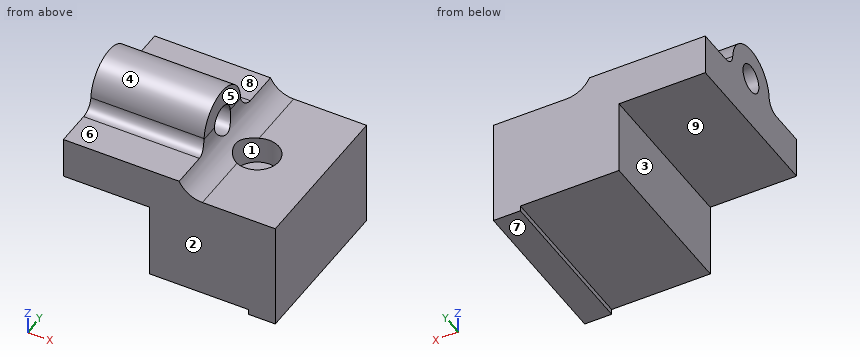
from build123d import *

# Parameters (mm, degrees)
PAD003_DEPTH         = 30
POCKET001_DEPTH      = 21.001
POCKET001_DEPTH_BACK = 18.286158
SKETCH010_R          = 2.6
POCKET002_DEPTH      = 21.001
POCKET002_DEPTH_BACK = 18.286158
SKETCH011_R          = 4
POCKET003_DEPTH      = 5
POCKET003_DEPTH_BACK = 100


with BuildPart() as part:
    # Sketch008 → Pad003 (new body)
    with BuildSketch(Plane.XZ):
        with BuildLine():
            Line((-16, 15), (0, 15))
            Line((0, 15), (0, 1))
            Line((0, 1), (18.285158, 1))
            Line((18.285158, 1), (18.285158, 0))
            Line((18.285158, 0), (23.285158, 0))
            Line((23.285158, 0), (23.285158, 20))
            Line((23.285158, 20), (9.7625, 20))
            ThreePointArc((5, 24.7625), (6.394904, 21.394904), (9.7625, 20))
            Line((5, 24.7625), (5, 30.6))
            Line((5, 30.6), (-16, 30.6))
            Line((-16, 30.6), (-16, 15))
        make_face()
    extrude(amount=PAD003_DEPTH)

    # Sketch009 (on Face1 of Pad003) → Pocket001 (cut, two sides)
    with BuildSketch(Plane(origin=(5, 0, 0), x_dir=(0, 0, 1), z_dir=(1, 0, 0))) as pocket001_sk:
        with BuildLine():
            ThreePointArc((24.943511, 9.009841), (30.6, 15), (24.943511, 20.990159))
            ThreePointArc((22.698592, 23.367503), (23.348515, 21.732615), (24.943511, 20.990159))
            Line((22.698592, 23.367503), (22.698592, 35))
            Line((22.698592, 35), (35.6, 35))
            Line((35.6, 35), (35.6, -5))
            Line((35.6, -5), (22.698592, -5))
            Line((22.698592, -5), (22.698592, 6.632497))
            ThreePointArc((24.943511, 9.009841), (23.348515, 8.267384), (22.698592, 6.632497))
        make_face()
    extrude(amount=-POCKET001_DEPTH, mode=Mode.SUBTRACT)
    extrude(pocket001_sk.sketch, amount=POCKET001_DEPTH_BACK, mode=Mode.SUBTRACT)

    # Sketch010 (on Face1 of Pocket001) → Pocket002 (cut, two sides)
    with BuildSketch(Plane(origin=(5, 0, 0), x_dir=(0, 0, 1), z_dir=(1, 0, 0))) as pocket002_sk:
        with Locations((24.6, 15)):
            Circle(SKETCH010_R)
    extrude(amount=-POCKET002_DEPTH, mode=Mode.SUBTRACT)
    extrude(pocket002_sk.sketch, amount=POCKET002_DEPTH_BACK, mode=Mode.SUBTRACT)

    # Sketch011 (on Face12 of Pocket002) → Pocket003 (cut, two sides)
    with BuildSketch(Plane(origin=(0, 0, 20), x_dir=(-1, 0, 0), z_dir=(0, 0, 1))) as pocket003_sk:
        with Locations((-11.47045, 15)):
            Circle(SKETCH011_R)
    extrude(amount=-POCKET003_DEPTH, mode=Mode.SUBTRACT)
    extrude(pocket003_sk.sketch, amount=POCKET003_DEPTH_BACK, mode=Mode.SUBTRACT)


solid = part.part
Input: part model. Units: mm. Frame: model coordinates. Face numbers are marked on the shaded views. A direction names the side the tool comes from. Give positions to 0.01 mm unless a question says otherwise; leave off trailing zeros. Write each loop counter-clockwise with the first axis right and the second up, starting at its lowest first coordinate (ties: lowest second). Pieces come first, ordered by that corner, then holes.
Q1. Pull-direction query (Y, two-part tool) for the marked faces 1, 2, 3 and 4; classes: pulls with the +Y half, pulls with the -Y half, needs draft (parallel to the pull), parting line crosses it, or undercut.
Q2. Section B-B, the plane y = -15. Output: boundary loops of the cut face in (x, z) (1 decimal).
Q3. Material intervals for probe 1 along X at (y, z) = (-15, 16); probe 2 along Z at (x, y) = (-5.5, -15); probe 3 along Z at (x, y) = (2.5, -6), sorted ascending.
Q4. First-contact query: P1, Ø1, axis at x = 10.5, y = -18, coming from the -Z side; P2, Ø4, axis at x = 11, y = -16.5, coming from the +Z side; P3, Ø13, axis at x = -11.5, y = -15, coming from the -Z side. Flat tips, straight axial feed; report the tip coordinate or a pass-through.
Q5. Section A-A, the plane x = -5. Output: boundary loops of the cut face in (y, z).
Q6. Set-up query: the marked faces 5, 6, 7, 8 and 9. Return all of +Z, -Z, +X, -X, +Y, -Y with unobstructed straight access to the full face (end or side cutting, diameter ignored); none if empty.
Q7. Section D-D, the plane z = 9. Output: boundary loops of the cut face in (x, y).
Q8. Section C-C, the plane y = -5. Output: boundary loops of the cut face in (x, z) (1 decimal).
Filled in:
1. face 1: undercut
1. face 2: pulls with the -Y half
1. face 3: needs draft
1. face 4: parting line crosses it
2. outline: (-16, 15) - (0, 15) - (0, 1) - (18.3, 1) - (18.3, 0) - (23.3, 0) - (23.3, 20) - (15.5, 20) - (15.5, 15) - (7.5, 15) - (7.5, 20.6) arc R4.8 cw to (5.9, 22) - (-16, 22) - close; (-16, 27.2) - (5, 27.2) - (5, 30.6) - (-16, 30.6) - close
3. probe 1: x = -16 to 7.47, 15.47 to 23.29
3. probe 2: z = 15 to 22, 27.2 to 30.6
3. probe 3: z = 1 to 22.7
4. P1: stops at z = 1
4. P2: stops at z = 15
4. P3: stops at z = 15
5. outline: (-30, 15) - (0, 15) - (0, 22.7) - (-6.63, 22.7) arc R2.38 cw to (-9.01, 24.94) arc R6 ccw to (-20.99, 24.94) arc R2.38 cw to (-23.37, 22.7) - (-30, 22.7) - close; hole circle Ø5.2 at (-15, 24.6)
6. face 5: +Z, +X, +Y, -Y
6. face 6: +Z, +X, -X, -Y
6. face 7: -Z, +X, -X, +Y, -Y
6. face 8: +Z, +X, -X, +Y
6. face 9: -Z, -X, +Y, -Y
7. outline: (0, -30) - (23.29, -30) - (23.29, 0) - (0, 0) - close
8. outline: (-16, 15) - (0, 15) - (0, 1) - (18.3, 1) - (18.3, 0) - (23.3, 0) - (23.3, 20) - (9.8, 20) arc R4.8 cw to (5.5, 22.7) - (-16, 22.7) - close
